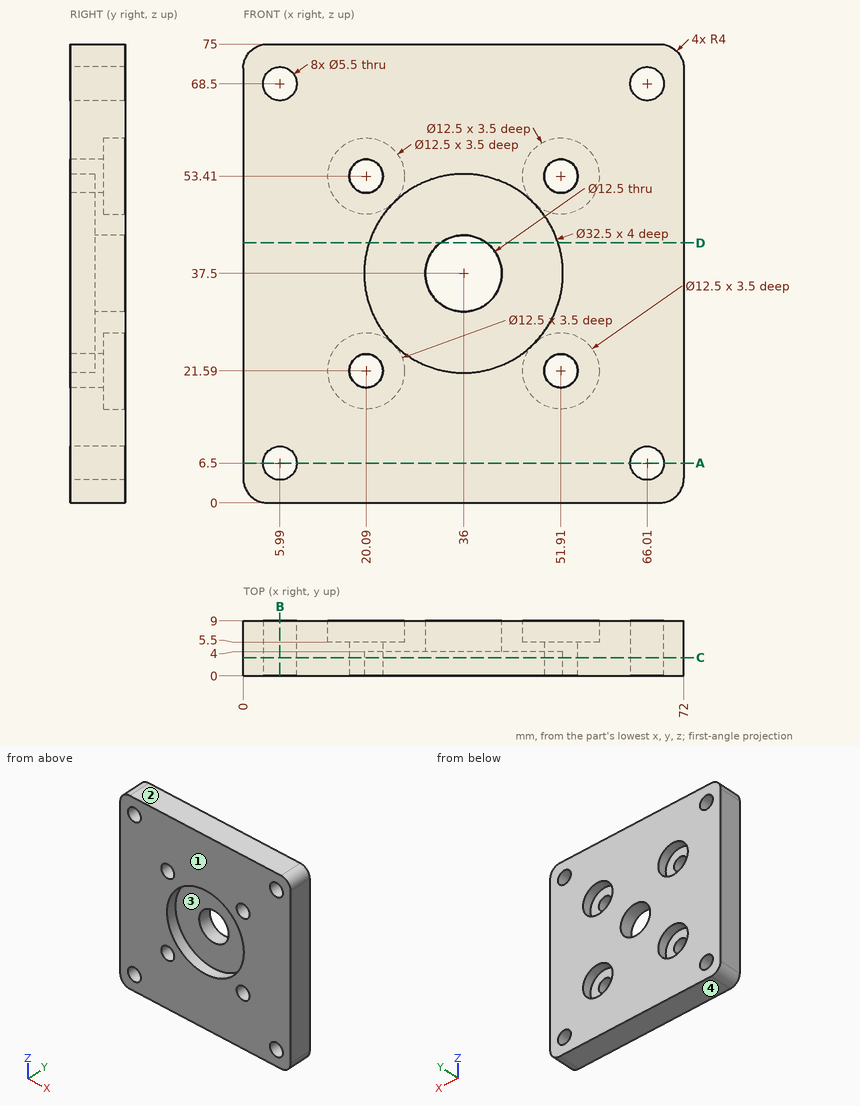
For this review, use the dimensioned drawing (mm, ordinates from the lowest corner) and the shaded views. Coordinates: 2 decimals unless noted, no trailing zeros. Loops run counter-clockwise (first coordinate to the right, second up) from the corner with the lowest first, then second, coordinate; pieces in that order, holes last. Notation, with made-up numbers: (82.5, 27.5) -> (93.5, 27.5) arc R17 cw to (93.5, 39.5) -> close; hole circle Ø11 at (76, 4.25). An arc over 180 degrees is marked (long way). Use a Markdown table: item, result. Add a question column.
1. Add section D-D on z = 42.5. Write out the cut boundary in (x, y).
2. Add section A-A on z = 6.5. Write out the cut boundary in (x, y), plus the area to 3 significant figures.
3. To check wall thickness, follow line 1 (Z direction, x = 52, y = 6.25); line 2 (X direction, y = 7.75, z = 37.5); line 3 (Z direction, x = 5.99, y = 3.5). State the ranges of each line that lie inside material, in increasing order.
4. Clearance check with flat-ended pins moving along their axes: pin 1 Ø4.5 at (x, z) = (20.09, 21.59) entering from -Y; pin 2 Ø6 at (x, z) = (22.5, 23.5) entering from +Y. State where each tip first meets the part, or that it passes through.
5. Add section B-B on x = 5.99. Write out the cut boundary in (y, z), plus the area to 3 significant figures.
6. Draft analysis for pull direction Z (two halves, no side actions). For the marked faces 1, 2, 3 and 4, state which applies: pulls with the +Z half, pulls with the -Z half, needs draft (parallel to the pull), parting line crosses it, or undercut.
7. Add section C-C on y = 3. Give the number of separate pieces and of enclosed holes in the cut face, plus the area to 3 significant figures.
Returned:
| question | item | result |
|---|---|---|
| 1 | outline | (0, 0) -> (20.54, 0) -> (20.54, 4) -> (32.25, 4) -> (32.25, 9) -> (0, 9) -> close; (39.75, 4) -> (51.46, 4) -> (51.46, 0) -> (72, 0) -> (72, 9) -> (39.75, 9) -> close |
| 2 | outline | (0, 0) -> (3.24, 0) -> (3.24, 9) -> (0, 9) -> close; (8.74, 0) -> (63.26, 0) -> (63.26, 9) -> (8.74, 9) -> close; (68.76, 0) -> (72, 0) -> (72, 9) -> (68.76, 9) -> close |
| 2 | area | 549 mm² |
| 3 | line 1 | z = 0 to 15.34, 27.84 to 47.16, 59.66 to 75 |
| 3 | line 2 | x = 0 to 29.75, 42.25 to 72 |
| 3 | line 3 | z = 0 to 3.75, 9.25 to 65.75, 71.25 to 75 |
| 4 | pin 1 | passes through |
| 4 | pin 2 | stops at y = 5.5 |
| 5 | outline | (0, 0) -> (9, 0) -> (9, 3.75) -> (0, 3.75) -> close; (0, 9.25) -> (9, 9.25) -> (9, 65.75) -> (0, 65.75) -> close; (0, 71.25) -> (9, 71.25) -> (9, 75) -> (0, 75) -> close |
| 5 | area | 576 mm² |
| 6 | face 1 | needs draft |
| 6 | face 2 | pulls with the +Z half |
| 6 | face 3 | undercut |
| 6 | face 4 | pulls with the -Z half |
| 7 | separate pieces | 1 |
| 7 | enclosed holes | 9 |
| 7 | area | 4,370 mm² |
